from build123d import *

# Parameters (mm, degrees)
SKETCH1_R           = 12.5
BOSS_EXTRUDE1_DEPTH = 50
SKETCH2_R           = 3.5
BOSS_EXTRUDE2_DEPTH = 2
SKETCH3_R           = 2
BOSS_EXTRUDE3_DEPTH = 11
SKETCH4_R           = 1.5
CUT_EXTRUDE1_DEPTH  = 5
SKETCH5_R           = 1
BOSS_EXTRUDE4_DEPTH = 11


with BuildPart() as part:
    # Sketch1 → Boss-Extrude1 (new body)
    with BuildSketch(Plane.XY):
        Circle(SKETCH1_R)
    extrude(amount=BOSS_EXTRUDE1_DEPTH)

    # Sketch2 → Boss-Extrude2 (add)
    with BuildSketch(Plane(origin=(0, 0, 0), x_dir=(-1, 0, 0), z_dir=(0, 0, -1))):
        Circle(SKETCH2_R)
    extrude(amount=BOSS_EXTRUDE2_DEPTH)

    # Sketch3 → Boss-Extrude3 (add)
    with BuildSketch(Plane(origin=(0, 0, -2), x_dir=(-1, 0, 0), z_dir=(0, 0, -1))):
        Circle(SKETCH3_R)
    extrude(amount=BOSS_EXTRUDE3_DEPTH)

    # Sketch4 → Cut-Extrude1 (cut)
    with BuildSketch(Plane(origin=(0, 0, 0), x_dir=(-1, 0, 0), z_dir=(0, 0, -1))):
        with Locations((-8.5, 0)):
            Circle(SKETCH4_R)
        with Locations((8.5, 0)):
            Circle(SKETCH4_R)
    extrude(amount=-CUT_EXTRUDE1_DEPTH, mode=Mode.SUBTRACT)

    # Sketch5 → Boss-Extrude4 (add)
    with BuildSketch(Plane.XY.offset(50)):
        Circle(SKETCH5_R)
    extrude(amount=BOSS_EXTRUDE4_DEPTH)


solid = part.part
Can you work these out from the model? Positions are in its coordinate system, mm. A direction names the side the tool comes from. Round coordinates to 2 decimals unless told otherwise and drop trailing zeros. Write each loop counter-clockwise with the first axis right and the second up, starting at its lowest first coordinate (ties: lowest second). Pieces come first, ordered by that corner, then holes. Notation, with made-up numbers: (16.5, 37) - (35.5, 37) arc R23 ccw to (35.5, 74) - close; hole circle Ø1 at (88.5, -18). An arc over 180 degrees is marked (long way). Write each question's results on one line, items separated by ' | '. Start each with the question number.
1) For pin 1 Ø3.5 at (x, y) = (-9, 0) entering from -Z; pin 2 Ø8 at (y, z) = (7.5, 36.5) entering from -X; pin 3 Ø1.8 at (x, y) = (8.5, 0) entering from -Z, each with a flat end and sliding along its axis, tell me the tip position at first contact or that it passes through.
2) Which directions (+Z, -Z, +X, -X, +Y, -Y) give clear straight access to the entire face, cutting with the end or side of a thin tool? Please do faces 4 (the cylindrical face through (10, 0, 2)), 5 (the cylindrical face through (0, -1, 55)), 6 (the flat face through (0, 0, -13)).
3) Suppose I cut it at A-A (y = 0). List the corners of the cut face in (x, z) for me.
4) Suppose I cut it at B-B (x = 0). List the corners of the cut face in (y, z) for me, and give its area (3 significant figures).
5) Suppose I cut it at C-C (z = 51). List the corners of the cut face in (x, y) for me, and give its area (3 significant figures).
6) We'd pull the mould along Y, two halves only. Please class faces 1 (the flat face through (3, -3, 0)), 2 (the flat face through (9, 0, 5)), 3 (the cylindrical face through (-3.233, -1.341, -0.986)): released by +Y, released by -Y, zero draft, split by the parting line, or undercut.
7) Please list where these lines run through material, in increasing order: line 1 (Z direction, x = 9, y = -2.75); line 2 (Y direction, x = 8.5, z = 2.25); line 3 (Z direction, x = -1.25, y = 1).
8) Suppose I cut it at D-D (x = -8). List the corners of the cut face in (y, z) for me, and give its area (3 significant figures).
Here are the results:
1) pin 1: stops at z = 0 | pin 2: stops at x = -12 | pin 3: stops at z = 5
2) face 4: -Z | face 5: +Z | face 6: -Z, +X, -X, +Y, -Y
3) outline: (-12.5, 0) - (-10, 0) - (-10, 5) - (-7, 5) - (-7, 0) - (-3.5, 0) - (-3.5, -2) - (-2, -2) - (-2, -13) - (2, -13) - (2, -2) - (3.5, -2) - (3.5, 0) - (7, 0) - (7, 5) - (10, 5) - (10, 0) - (12.5, 0) - (12.5, 50) - (1, 50) - (1, 61) - (-1, 61) - (-1, 50) - (-12.5, 50) - close
4) outline: (-12.5, 0) - (-3.5, 0) - (-3.5, -2) - (-2, -2) - (-2, -13) - (2, -13) - (2, -2) - (3.5, -2) - (3.5, 0) - (12.5, 0) - (12.5, 50) - (1, 50) - (1, 61) - (-1, 61) - (-1, 50) - (-12.5, 50) - close | area: 1,330 mm2
5) outline: circle Ø2 at (0, 0) | area: 3.14 mm2
6) face 1: zero draft | face 2: undercut | face 3: split by the parting line
7) line 1: z = 0 to 50 | line 2: y = -9.17 to -1.5, 1.5 to 9.17 | line 3: z = -13 to 50
8) outline: (-9.6, 0) - (-1.41, 0) - (-1.41, 5) - (1.41, 5) - (1.41, 0) - (9.6, 0) - (9.6, 50) - (-9.6, 50) - close | area: 946 mm2
